Design review of the part built by this model. Coordinates are the model's own, in mm. A direction names the side the tool comes from. Give positions to 0.01 mm unless a question says otherwise; leave off trailing zeros. Write each loop counter-clockwise with the first axis right and the second up, starting at its lowest first coordinate (ties: lowest second). Pieces come first, ordered by that corner, then holes.
```python
from build123d import *

# Parameters (mm, degrees)
SKETCH1_W           = 85
SKETCH1_H           = 95
BOSS_EXTRUDE1_DEPTH = 7
SKETCH2_W           = 30
SKETCH2_H           = 30
CUT_EXTRUDE1_DEPTH  = 7
SKETCH4_R           = 1.5
CUT_EXTRUDE2_DEPTH  = 10.5
SKETCH6_R           = 1.5
CUT_EXTRUDE3_DEPTH  = 8
CUT_EXTRUDE4_DEPTH  = 10
SKETCH8_R           = 1.5
CUT_EXTRUDE5_DEPTH  = 10
CUT_EXTRUDE6_DEPTH  = 5
SKETCH11_R          = 1.5
CUT_EXTRUDE8_DEPTH  = 4
SKETCH12_W          = 22
SKETCH12_H          = 32
CUT_EXTRUDE9_DEPTH  = 10
SKETCH13_W          = 31.5
SKETCH13_H          = 7
SKETCH13_R          = 1.5
CUT_EXTRUDE10_DEPTH = 0.5


with BuildPart() as part:
    # Sketch1 → Boss-Extrude1 (new body)
    with BuildSketch(Plane.XY):
        with Locations((42.5, 47.5)):
            Rectangle(SKETCH1_W, SKETCH1_H)
    extrude(amount=BOSS_EXTRUDE1_DEPTH)

    # Sketch2 → Cut-Extrude1 (cut)
    with BuildSketch(Plane.XY.offset(7)):
        with Locations((42.5, 45)):
            Rectangle(SKETCH2_W, SKETCH2_H)
    extrude(amount=-CUT_EXTRUDE1_DEPTH, mode=Mode.SUBTRACT)

    # Sketch4 → Cut-Extrude2 (cut)
    with BuildSketch(Plane(origin=(0, 95, 0), x_dir=(1, 0, 0), z_dir=(0, 1, 0))):
        with Locations((21.25, -3.5)):
            Circle(SKETCH4_R)
        with Locations((63.75, -3.5)):
            Circle(SKETCH4_R)
    extrude(amount=-CUT_EXTRUDE2_DEPTH, mode=Mode.SUBTRACT)

    # Sketch6 → Cut-Extrude3 (cut)
    with BuildSketch(Plane(origin=(0, 0, 0), x_dir=(-1, 0, 0), z_dir=(0, 0, -1))):
        with Locations((-80.75, 90.75)):
            Circle(SKETCH6_R)
        with Locations((-4.25, 90.75)):
            Circle(SKETCH6_R)
        with Locations((-4.45, 4.25)):
            Circle(SKETCH6_R)
        with Locations((-80.75, 7.25)):
            Circle(SKETCH6_R)
    extrude(amount=-CUT_EXTRUDE3_DEPTH, mode=Mode.SUBTRACT)

    # Sketch7 → Cut-Extrude4 (cut)
    with BuildSketch(Plane(origin=(0, 0, 0), x_dir=(-1, 0, 0), z_dir=(0, 0, -1))):
        with BuildLine():
            Line((-85, 45), (-85, 0))
            Line((-85, 0), (0, 0))
            Line((0, 0), (0, 45))
            ThreePointArc((0, 45), (-42.5, 2.5), (-85, 45))
        make_face()
    extrude(amount=-CUT_EXTRUDE4_DEPTH, mode=Mode.SUBTRACT)

    # Sketch8 → Cut-Extrude5 (cut)
    with BuildSketch(Plane.XY.offset(7)):
        with Locations((80.75, 63)):
            Circle(SKETCH8_R)
        with Locations((4.25, 63)):
            Circle(SKETCH8_R)
    extrude(amount=-CUT_EXTRUDE5_DEPTH, mode=Mode.SUBTRACT)

    # Sketch9 → Cut-Extrude6 (cut)
    with BuildSketch(Plane(origin=(0, 0, 0), x_dir=(-1, 0, 0), z_dir=(0, 0, -1))):
        Polygon((-79.045, 65.953146627), (-82.455, 65.953146627), (-84.16, 63), (-82.455, 60.046853373), (-79.045, 60.046853373), (-77.34, 63), align=None)
        Polygon((-0.84, 63), (-2.545, 60.046853373), (-5.955, 60.046853373), (-7.66, 63), (-5.955, 65.953146627), (-2.545, 65.953146627), align=None)
    extrude(amount=-CUT_EXTRUDE6_DEPTH, mode=Mode.SUBTRACT)

    # Sketch11 → Cut-Extrude8 (cut)
    with BuildSketch(Plane.XY.offset(7)):
        with Locations((42.5, 6.75)):
            Circle(SKETCH11_R)
    extrude(amount=-CUT_EXTRUDE8_DEPTH, mode=Mode.SUBTRACT)

    # Sketch12 → Cut-Extrude9 (cut)
    with BuildSketch(Plane(origin=(0, 0, 0), x_dir=(-1, 0, 0), z_dir=(0, 0, -1))):
        with Locations((-42.5, 79)):
            Rectangle(SKETCH12_W, SKETCH12_H)
    extrude(amount=-CUT_EXTRUDE9_DEPTH, mode=Mode.SUBTRACT)

    # Sketch13 → Cut-Extrude10 (cut)
    with BuildSketch(Plane(origin=(0, 95, 0), x_dir=(1, 0, 0), z_dir=(0, 1, 0))):
        with Locations((15.75, -3.5)):
            Rectangle(SKETCH13_W, SKETCH13_H)
        with Locations((21.25, -3.5)):
            Circle(SKETCH13_R, mode=Mode.SUBTRACT)
        with Locations((69.25, -3.5)):
            Rectangle(SKETCH13_W, SKETCH13_H)
        with Locations((63.75, -3.5)):
            Circle(SKETCH13_R, mode=Mode.SUBTRACT)
    extrude(amount=-CUT_EXTRUDE10_DEPTH, mode=Mode.SUBTRACT)


solid = part.part
```
(1) Clearance check with flat-ended pins moving along their axes: P1, Ø2, axis at x = 42, z = 4.5, coming from the +Y side; P2, Ø2.5, axis at x = 4.25, y = 90.75, coming from the -Z side; P3, Ø1.8, axis at x = 21.25, z = 3.5, coming from the +Y side; P4, Ø4, axis at x = 80, z = 1.5, coming from the -Y side. State where each tip first meets the part, or that it passes through.
Resolved:
P1: stops at y = 63
P2: passes through
P3: stops at y = 84.5
P4: stops at y = 21.63
(2) Consider section C-C, the plane y = 40. Give the boundary of the cut face in (x, z).
Resolved:
outline: (0.3, 0) - (27.5, 0) - (27.5, 7) - (0.3, 7) - close; (57.5, 0) - (84.7, 0) - (84.7, 7) - (57.5, 7) - close
(3) Mouldability with a two-part tool opening along Y and no side actions: class faces 1 (the face through (69, 94.5, 3)), 2 (the face through (1.704, 64.497, 2.465)), 3 (the face through (1.681, 61.544, 2.465)), 4 (the face through (53.5, 79, 3)) as pulls with the +Y half, pulls with the -Y half, needs draft (parallel to the pull), parting line crosses it, or undercut.
Resolved:
face 1: pulls with the +Y half
face 2: undercut
face 3: undercut
face 4: needs draft
(4) To check wall thickness, follow L1, parallel to X at y = 87.5, z = 3.5; L2, parallel to X at y = 36.5, z = 0.5; L3, parallel to X at y = 77, z = 3. State the ranges of each line that lie inside material, in increasing order.
Resolved:
L1: x = 0 to 19.75, 22.75 to 31.5, 53.5 to 62.25, 65.25 to 85
L2: x = 0.86 to 27.5, 57.5 to 84.14
L3: x = 0 to 31.5, 53.5 to 85
(5) Consider section A-A, the plane y = 90.75. Give the boundary of the cut face in (x, z).
Resolved:
outline: (0, 0) - (2.75, 0) - (2.75, 7) - (0, 7) - close; (5.75, 0) - (31.5, 0) - (31.5, 7) - (5.75, 7) - close; (53.5, 0) - (79.25, 0) - (79.25, 7) - (53.5, 7) - close; (82.25, 0) - (85, 0) - (85, 7) - (82.25, 7) - close; hole circle Ø3 at (21.25, 3.5); hole circle Ø3 at (63.75, 3.5)
(6) Tool access review of faces 5 (the face through (6.796, 61.503, 2.465)), 6 (the face through (42, 30, 4)), 7 (the face through (42, 7, 3)): name each direction out of +Z, -Z, +X, -X, +Y, -Y from which nothing blocks a thin tool from reaching the whole face with its end or side.
Resolved:
face 5: -Z
face 6: +Z, -Z
face 7: +Z
(7) Consider section D-D, the plane x = 80.75. Give the boundary of the cut face in (y, z).
Resolved:
outline: (26.47, 0) - (60.05, 0) - (60.05, 5) - (61.5, 5) - (61.5, 7) - (26.47, 7) - close; (64.5, 5) - (65.95, 5) - (65.95, 0) - (89.25, 0) - (89.25, 7) - (64.5, 7) - close; (92.25, 0) - (94.5, 0) - (94.5, 7) - (92.25, 7) - close
(8) Consider section B-B, the plane x = 42.5. Give the boundary of the cut face in (y, z).
Resolved:
outline: (2.5, 0) - (30, 0) - (30, 7) - (8.25, 7) - (8.25, 3) - (5.25, 3) - (5.25, 7) - (2.5, 7) - close; (60, 0) - (63, 0) - (63, 7) - (60, 7) - close
